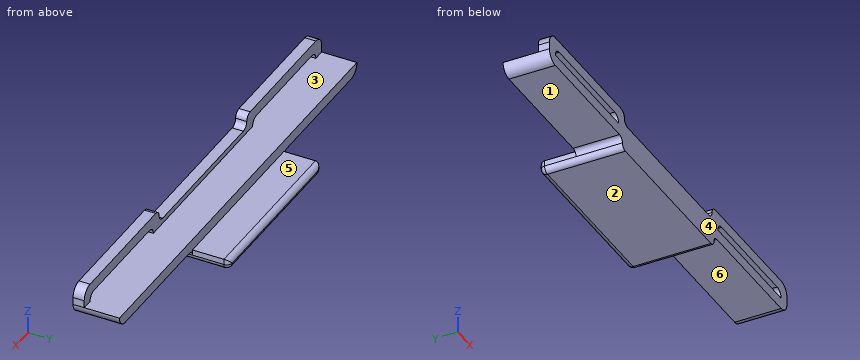
```python
from build123d import *

# Parameters (mm, degrees)
F1_DEPTH = 6
F2_DEPTH = 25
F0_W     = 94
F0_H     = 6
F3_DEPTH = 45
F4_W     = 65
F4_H     = 4
F5_DEPTH = 25
F6_R     = 3.99999
F7_R     = 3.49999
F8_R     = 5.99999
F9_R     = 2.99999


# Not quite as in the source:
# - two fillets or chamfers of one size are made in one step
# - a fillet or chamfer is up to 0.001 mm smaller than in the source, because OpenCascade refuses the exact size


with BuildPart() as f1:
    # F0 (on Front) → F1 (new body)
    with BuildSketch(Plane.XZ):
        Polygon((-122, 22), (-122, 12), (122, 12), (122, 22), (45, 22), (45, 15), (-45, 15), (-45, 22), align=None)
    extrude(amount=-F1_DEPTH)

    # F0 (on Front) → F2 (join)
    with BuildSketch(Plane.XZ):
        Polygon((-122, 12), (-122, 6), (-47, 6), (47, 6), (122, 6), (122, 12), align=None)
    extrude(amount=-F2_DEPTH)

    # F0 (on Front) → F3 (join, through all)
    with BuildSketch(Plane.XZ):
        with Locations((0, 3)):
            Rectangle(F0_W, F0_H)
    extrude(amount=-F3_DEPTH)

    # F4 (on face) → F5 (cut)
    with BuildSketch(Plane(origin=(0, 6, 0), x_dir=(-1, 0, 0), z_dir=(0, 1, 0))):
        with Locations((83.5, 14)):
            Rectangle(F4_W, F4_H)
        with Locations((-83.5, 14)):
            Rectangle(F4_W, F4_H)
    extrude(amount=-F5_DEPTH, mode=Mode.SUBTRACT)

    # F6 (radius 4 in the source; OpenCascade refuses exactly that, so slightly less here)
    f6_edges = [f1.edges().sort_by_distance(p)[0] for p in [
        (-51, 3, 16),
        (-116, 3, 16),
        (51, 3, 16),
        (116, 3, 16),
    ]]
    fillet(f6_edges, radius=F6_R)

    # F7 (radius 3.5 in the source; OpenCascade refuses exactly that, so slightly less here)
    f7_edges = [f1.edges().sort_by_distance(p)[0] for p in [
        (-45, 3, 15),
        (-45, 3, 22),
        (45, 3, 15),
        (45, 3, 22),
    ]]
    fillet(f7_edges, radius=F7_R)

    # F8 (radius 6 in the source; OpenCascade refuses exactly that, so slightly less here)
    f8_edges = [f1.edges().sort_by_distance(p)[0] for p in [
        (-122, 3, 22),
        (122, 3, 22),
        (-122, 12.5, 6),
        (122, 12.5, 6),
    ]]
    fillet(f8_edges, radius=F8_R)

    # F9 (radius 3 in the source; OpenCascade refuses exactly that, so slightly less here)
    f9_edges = [f1.edges().sort_by_distance(p)[0] for p in [
        (47, 12.5, 6),
        (47, 22.5, 0),
        (-47, 22.5, 0),
        (-47, 12.5, 6),
        (-47, 45, 3),
        (0, 45, 0),
        (47, 45, 3),
        (0, 45, 6),
    ]]
    fillet(f9_edges, radius=F9_R)


solid = f1.part
```
Build history of the part. All positions in model axes, mm. Face numbers are marked on the shaded views. A direction names the side the tool comes from. Round coordinates to 2 decimals unless told otherwise and drop trailing zeros. Write each loop counter-clockwise with the first axis right and the second up, starting at its lowest first coordinate (ties: lowest second). Pieces come first, ordered by that corner, then holes.
1) Band-saw the part on D-D, the plane y = 35.5. List the corners of the cut face in (x, z), and give its area (3 significant figures).
2) 3-axis set-ups, long thin cutter, end or side, ignore diameter. For the marked faces 1 and 2: which of +Z, -Z, +X, -X, +Y, -Y reach the whole face in a straight line?
3) Band-saw the part on A-A, the plane x = -60.5. List the corners of the cut face in (y, z), and give its area (3 significant figures).
4) Pin check, flat tips, straight feed: pin 1 (0.9 mm diameter, centred on y = 29, z = 4, fed in from +X); pin 2 (13.5 mm diameter, centred on x = -11, y = 34, fed in from +Z); pin 3 (4 mm diameter, centred on x = -69.5, y = 9, fed in from +Z). Stop position of each tip, or through.
5) Mould opens along Z. For the marked faces 3, 4, 5 and 6 say: +Z half, -Z half, draft (parallel to the pull), parting line (faces both ways), or undercut.
6) Drill centre lines: probe 1 along X at (y, z) = (4, 12.5); probe 2 along X at (y, z) = (29.5, 3); probe 3 along Y at (x, z) = (-5, 6.5). Where is each one in solid material? Low to high.
Ans:
1. outline: (-47, 3) arc R3 ccw to (-44, 0) - (44, 0) arc R3 ccw to (47, 3) - (47, 6) - (-47, 6) - close
1. area: 560 mm2
2. face 1: -Z, -X, +Y, -Y
2. face 2: -Z, +X, -X, +Y, -Y
3. outline: (0, 6) - (25, 6) - (25, 12) - (0, 12) - close; (0, 16) - (6, 16) - (6, 22) - (0, 22) - close
3. area: 186 mm2
4. pin 1: stops at x = 47
4. pin 2: stops at z = 6
4. pin 3: stops at z = 12
5. face 3: undercut
5. face 4: draft
5. face 5: +Z half
5. face 6: -Z half
6. probe 1: x = -122 to -115.97, -51.03 to 51.03, 115.97 to 122
6. probe 2: x = -47 to 47
6. probe 3: y = 0 to 25
